```python
from build123d import *

# Parameters (mm, degrees)
BASENUT_START = -2.9
BASENUTSKE_R  = 1.25
BASENUT_DEPTH = 2.9


# Read off the part's stored shape, not the designer's step: ThreadSchematic
with BuildPart() as part:
    # BaseNutSke → BaseNut (new body)
    with BuildSketch(Plane.XY.offset(BASENUT_START)):
        Polygon((2.75, 1.58771324), (2.75, -1.58771324), (0, -3.175426481), (-2.75, -1.58771324), (-2.75, 1.58771324), (0, 3.175426481), align=None)
        Circle(BASENUTSKE_R, mode=Mode.SUBTRACT)
    extrude(amount=BASENUT_DEPTH)

    # Sketch5 (on Front Plane) → EndChamfer (revolve, cut)
    with BuildSketch(Plane.XY):
        Polygon((2.8746, 1.5), (2.682042927, 1.225), (2.9254, 1.225), (2.9254, 1.5), align=None)
    revolve(axis=Axis((2.9254, 1.225, 0), (-1, 0, 0)), mode=Mode.SUBTRACT)

    # Sketch3 → Double-Chamfer (revolve, cut)
    with BuildSketch(Plane(origin=(0, 0, 0), x_dir=(0, 0, -1), z_dir=(1, 0, 0))):
        Polygon((2.9, 2.75), (2.654379907, 3.175426481), (2.654379907, 13.175426481), (12.9, 13.175426481), (12.9, 2.75), align=None)
        Polygon((0.245620093, 13.175426481), (-10, 13.175426481), (-10, 2.75), (0, 2.75), (0.245620093, 3.175426481), align=None)
    revolve(axis=Axis((0, 0, 0), (0, 0, -1)), mode=Mode.SUBTRACT)

    # ThreadSchematic outline → ThreadSchematic (revolve, cut)
    with BuildSketch(Plane.XZ):
        Polygon((1.25, 0), (1.25, -0.175051885), (1.5, 0), align=None)
        Polygon((1.5, -2.8746), (1.25, -2.699548115), (1.25, -2.9), (1.5, -2.9), align=None)
    revolve(axis=Axis((0, 0, 0), (0, 0, 1)), mode=Mode.SUBTRACT)


solid = part.part
```
The listing builds one solid part. Answer for the finished solid, in the listing's coordinates (mm). Give positions to 0.01 mm unless a question says otherwise; leave off trailing zeros. Order: outer loops, then holes, each group sorted by start corner. A loop starts at its lowest first (then second) coordinate and runs counter-clockwise, first axis right, second up. Notation, with made-up numbers: (50.25, 15) -> (104.25, 15) arc R7 ccw to (104.25, 19) -> close; hole circle Ø11 at (-26.75, 68.5). An arc over 180 degrees is marked (long way). Answer as CSV lines item,"result". Start each with the question number.
Q1. Determine the mould class of faces 1 (the flat face through (-1.2, -1.2, 0)), 2 (the conical face through (-2.52, 1.44, -0.09)), 3 (the flat face through (1.394, -2.37, -1.47)), 4 (the cylindrical face through (-0.27, -1.22, -1.45)) for opening direction X: pulls with the +X half, pulls with the -X half, needs draft (parallel to the pull), parting line crosses it, or undercut.
Q2. Find the intervals of material crossed by L1, parallel to X at y = 0.25, z = -1.2; L2, parallel to Y at x = -0.35, z = -0.2; L3, parallel to X at y = 1, z = -0.95, in increasing order.
Q3. A cutting plane is placed at A-A (z = -2.35). Determine the outline of the cut face in (x, y).
Q4. Given pin 1 (1.5 mm diameter, centred on x = -1.5, z = -1.5, fed in from -Y), flat-ended and moving along its own axis, determine where the tip first touches the part or whether it passes through.
Results found:
1,face 1,"needs draft"
1,face 2,"pulls with the -X half"
1,face 3,"pulls with the +X half"
1,face 4,"undercut"
2,L1,"-2.75 to -1.22, 1.22 to 2.75"
2,L2,"-2.97 to -1.2, 1.2 to 2.97"
2,L3,"-2.75 to -0.75, 0.75 to 2.75"
3,outline,"(-2.75, -1.59) -> (0, -3.18) -> (2.75, -1.59) -> (2.75, 1.59) -> (0, 3.18) -> (-2.75, 1.59) -> close; hole circle Ø2.5 at (0, 0)"
4,pin 1,"y = -2.74"
